Check sheet for the drawn part. Datum: minimum x, y, z corner. Units: mm. Round coordinates to 2 decimals unless told otherwise and drop trailing zeros. Loops run counter-clockwise (first coordinate to the right, second up) from the corner with the lowest first, then second, coordinate; pieces in that order, holes last. Notation, with made-up numbers: (-40, -36.5) -> (-34, -36.5) arc R18 cw to (-34, -8.5) -> close; hole circle Ø1 at (-26, 7.5). An arc over 180 degrees is marked (long way). Return JSON: item names as keys, results as strings.
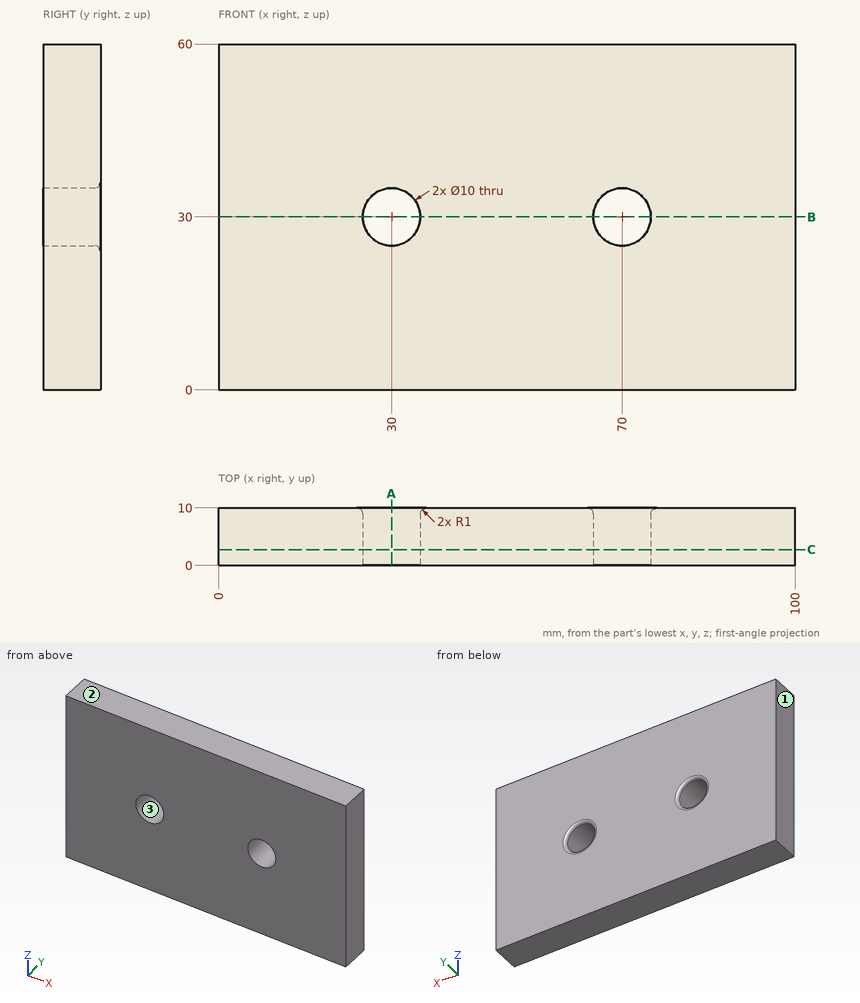
Q1. Draft check along Z on the marked faces 1, 2 and 3. Enter one of: released by +Z, released by -Z, zero draft, split by the parting line, or undercut.
Results list:
{"face 1": "zero draft", "face 2": "released by +Z", "face 3": "undercut"}
Q2. Go/stop test with a flat-tipped pin: pin 1 (6 mm diameter, centred on x = 12, z = 52, fed in from -Y). Record where the tip stops, or that it passes through.
Results list:
{"pin 1": "y = 0"}
Q3. Material ranges on line 1 (Z direction, x = 30, y = 4.75); line 2 (X direction, y = 3, z = 30); line 3 (X direction, y = 8, z = 29), recorded low to high.
Results list:
{"line 1": "0 to 25, 35 to 60", "line 2": "0 to 25, 35 to 65, 75 to 100", "line 3": "0 to 25.1, 34.9 to 65.1, 74.9 to 100"}
Q4. Section check B-B (z = 30). Record the boundary of the cut face in (x, y).
Results list:
{"outline": "(0, 0) -> (25, 0) -> (25, 9) arc R1 ccw to (24, 10) -> (0, 10) -> close; (35, 0) -> (65, 0) -> (65, 9) arc R1 ccw to (64, 10) -> (36, 10) arc R1 ccw to (35, 9) -> close; (75, 0) -> (100, 0) -> (100, 10) -> (76, 10) arc R1 ccw to (75, 9) -> close"}
Q5. Section check A-A (x = 30). Record the boundary of the cut face in (y, z), then the cut area to 3 significant figures.
Results list:
{"outline": "(0, 0) -> (10, 0) -> (10, 24) arc R1 ccw to (9, 25) -> (0, 25) -> close; (0, 35) -> (9, 35) arc R1 ccw to (10, 36) -> (10, 60) -> (0, 60) -> close", "area": "500 mm^2"}
Q6. Section check C-C (y = 2.75). Record the boundary of the cut face in (x, z).
Results list:
{"outline": "(0, 0) -> (100, 0) -> (100, 60) -> (0, 60) -> close; hole circle Ø10 at (30, 30); hole circle Ø10 at (70, 30)"}
